Input: part model. Units: mm. Frame: model coordinates. Face numbers are marked on the shaded views. A direction names the side the tool comes from. Round coordinates to 2 decimals unless told otherwise and drop trailing zeros. Loops run counter-clockwise (first coordinate to the right, second up) from the corner with the lowest first, then second, coordinate; pieces in that order, holes last. Notation, with made-up numbers: (86.25, 79.5) -> (139.25, 79.5) arc R29 cw to (139.25, 110.5) -> close; hole circle Ø1 at (-40, -1). An arc over 180 degrees is marked (long way). Answer as a JSON object with one key per item and string values. Group by question number.
Item 1: Material intervals for line 1 (X direction, y = 8.75, z = 11.75); line 2 (Z direction, x = 6, y = 2.25); line 3 (X direction, y = -2.5, z = 5), sorted ascending. Write a range as [from, to].
Item 2: Section query D-D on x = 3.5. Return loops of the section in (y, z) (3 decimals).
Item 3: Section query B-B on x = 5. Return loops of the section in (y, z) (3 decimals), and give its area (3 significant figures).
Item 4: Section query A-A on y = 4.5. Return loops of the section in (x, z) (3 decimals), and give its area (3 significant figures).
Item 5: Draft query along Y for the marked faces 1, 2, 3 and 4. Return one class per face: released by +Y, released by -Y, zero draft, split by the parting line, or undercut.
Item 6: Pin query (flat end, axial travel): pin 1 (4.5 mm diameter, centred on y = 0, z = 19, fed in from -X); pin 2 (1.6 mm diameter, centred on x = 1.5, y = -4, fed in from +Z). Return the tip coordinate at first contact, or that it passes through.
Item 7: Section query C-C on z = 9.25. Return loops of the section in (x, y), and give its area (3 significant figures).
Item 8: Set-up query: the marked faces 5 and 6. Return all of +Z, -Z, +X, -X, +Y, -Y with unobstructed straight access to the full face (end or side cutting, diameter ignored); none if empty.
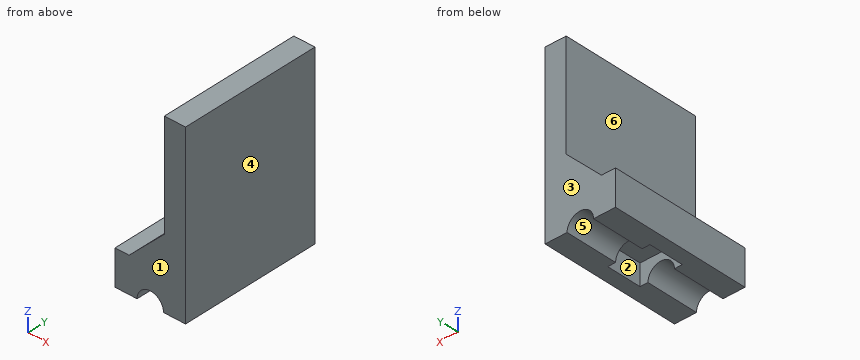
from build123d import *

# Parameters (mm, degrees)
BOSS_EXTRUDE1_DEPTH     = 10
CUT_EXTRUDE2_DEPTH      = 4.88
CUT_EXTRUDE4_DEPTH      = 18.67766953
CUT_EXTRUDE4_DEPTH_BACK = 18.67766953
SKETCH6_3_R             = 1.875
CUT_EXTRUDE5_DEPTH      = 24.58495283
CUT_EXTRUDE5_DEPTH_BACK = 24.58495283
SKETCH7_OUTSIDE_W       = 17.386
SKETCH7_OUTSIDE_H       = 22.386
SKETCH8_W               = 3
SKETCH8_H               = 20
BOSS_EXTRUDE2_DEPTH     = 20
CHAMFER1_SIZE           = 5


with BuildPart() as part:
    # Sketch2 → Boss-Extrude1 (new body)
    with BuildSketch(Plane.YZ):
        Polygon((-10, -7.5), (-4, -7.5), (-5, -5.5), (-2.5, -5.5), (-2.5, -3), (2.5, -3), (2.5, -5.5), (5, -5.5), (4, -7.5), (10, -7.5), (10, 7.5), (-10, 7.5), align=None)
    extrude(amount=BOSS_EXTRUDE1_DEPTH)

    # Sketch4 → Cut-Extrude2 (cut)
    with BuildSketch(Plane(origin=(0, 0, -3), x_dir=(1, 0, 0), z_dir=(0, 0, -1))):
        Polygon((5, 2.5), (2, 2.5), (2, -2.5), (8, -2.5), (8, 2.5), align=None)
    extrude(amount=-CUT_EXTRUDE2_DEPTH, mode=Mode.SUBTRACT)

    # Sketch6_3 → Cut-Extrude4 (cut, two sides: drawn at the far end of the back side and taken through both)
    with BuildSketch(Plane.XZ.offset(-2.5).offset(-CUT_EXTRUDE4_DEPTH_BACK)):
        with Locations(Location((5, -1.12, 0), (0, 0, 270))):
            Circle(SKETCH6_3_R)
    extrude(amount=CUT_EXTRUDE4_DEPTH + CUT_EXTRUDE4_DEPTH_BACK, mode=Mode.SUBTRACT)

    # Sketch7 outside → Cut-Extrude5 (cut, two sides: drawn at the far end of the back side and taken through both)
    with BuildSketch(Plane(origin=(0, 10, 0), x_dir=(-1, 0, 0), z_dir=(0, 1, 0)).offset(-CUT_EXTRUDE5_DEPTH_BACK)):
        with Locations((-5, 0)):
            Rectangle(SKETCH7_OUTSIDE_W, SKETCH7_OUTSIDE_H)
        with BuildLine():
            Line((-10, -1.12), (-6.875, -1.12))
            ThreePointArc((-6.875, -1.12), (-5, 0.755), (-3.125, -1.12))
            Line((-3.125, -1.12), (0, -1.12))
            Line((0, -1.12), (0, 3.88))
            Line((0, 3.88), (-10, 3.88))
            Line((-10, 3.88), (-10, -1.12))
        make_face(mode=Mode.SUBTRACT)
    extrude(amount=CUT_EXTRUDE5_DEPTH + CUT_EXTRUDE5_DEPTH_BACK, mode=Mode.SUBTRACT)

    # Sketch8 → Boss-Extrude2 (add)
    with BuildSketch(Plane.XY.offset(3.88)):
        with Locations((8.5, 0)):
            Rectangle(SKETCH8_W, SKETCH8_H)
    extrude(amount=BOSS_EXTRUDE2_DEPTH)

    # Chamfer1
    chamfer1_edges = [part.edges().sort_by_distance(p)[0] for p in [
        (7, 0, 3.88),
    ]]
    chamfer(chamfer1_edges, length=CHAMFER1_SIZE)


solid = part.part
Solved:
{
 "1": {"line 1": "[7, 10]", "line 2": "[1.88, 7.88]", "line 3": "[3.12, 10]"},
 "2": {"outline": "(-10, 0.005) -> (-2.5, 0.005) -> (-2.5, 1.88) -> (2.5, 1.88) -> (2.5, 0.005) -> (10, 0.005) -> (10, 5.38) -> (-10, 5.38) -> close"},
 "3": {"outline": "(-10, 0.755) -> (-2.5, 0.755) -> (-2.5, 1.88) -> (2.5, 1.88) -> (2.5, 0.755) -> (10, 0.755) -> (10, 6.88) -> (-10, 6.88) -> close", "area": "117 mm²"},
 "4": {"outline": "(0, -1.12) -> (3.125, -1.12) arc R1.875 cw to (6.875, -1.12) -> (10, -1.12) -> (10, 23.88) -> (7, 23.88) -> (7, 8.88) -> (2, 3.88) -> (0, 3.88) -> close", "area": "117 mm²"},
 "5": {"face 1": "released by -Y", "face 2": "undercut", "face 3": "released by +Y", "face 4": "zero draft"},
 "6": {"pin 1": "x = 7", "pin 2": "z = 4.18"},
 "7": {"outline": "(7, -10) -> (10, -10) -> (10, 10) -> (7, 10) -> close", "area": "60.0 mm²"},
 "8": {"face 5": "-Z, +Y, -Y", "face 6": "+Z, -X, +Y, -Y"}
}
